Read the model definition and answer for the solid it produces. Units are mm, in the model's axes. Round coordinates to 2 decimals unless told otherwise and drop trailing zeros. Order: outer loops, then holes, each group sorted by start corner. A loop starts at its lowest first (then second) coordinate and runs counter-clockwise, first axis right, second up. Notation, with made-up numbers: (61.25, -15) -> (68.25, -15) arc R12 cw to (68.25, -4) -> close; hole circle Ø5 at (89, 68.25). An arc over 180 degrees is marked (long way). One line per item, written item: value. Start each with the question number.
1. Section D-D (z = 23.5) is taken. Give the vertices of the cut face in (x, y), then the cut area to 3 significant figures.
2. Flat-ended cylindrical pins translate along their axes: pin 1 Ø4 at (x, z) = (31, 16) entering from -Y; pin 2 Ø1 at (x, z) = (14.5, 9.5) entering from -Y; pin 3 Ø4 at (x, z) = (48.5, 13) entering from -Y; pin 4 Ø2 at (x, y) = (8, -2) entering from +Z. Find the tip coordinate at first contact, or state that the pin passes through.
3. Section A-A (z = 17.5) is taken. Give the vertices of the cut face in (x, y), then the cut area to 3 significant figures.
4. The mould has two halves that part along Y. Classify faces 1 (the face through (12, 0, 13)), 2 (the face through (17.334, 13.791, 23.872)), 3 (the face through (0, 8, 13)): released by +Y, released by -Y, zero draft, split by the parting line, or undercut.
5. Section C-C (y = -6.75) is taken. Give the vertices of the cut face in (x, z).
6. Section B-B (x = 10) is taken. Give the vertices of the cut face in (y, z).
7. Consider line 1 (Y direction, x = 2.5, z = 14); line 2 (Y direction, x = 51, z = 6.75); line 3 (X direction, y = 6.5, z = 19.75). Determine where each line is inside the solid, lowest interval first.
from build123d import *

# Parameters (mm, degrees)
F1_DEPTH = 25.4
F2_R     = 5.08
F3_R     = 5.08


# Not quite as in the source:
# - a feature names something its author has since deleted; it is built from what else it names


with BuildPart() as f1:
    # F0 (on Top) → F1 (new body)
    with BuildSketch(Plane.XY):
        Polygon((0, 15.24), (0, 0), (24.13, 0), (55.0936062386, -11.4706359327), (30.48, 15.24), align=None)
    extrude(amount=F1_DEPTH)

    # F2
    f2_edges = [f1.edges().sort_by_distance(p)[0] for p in [
        (15.24, 15.24, 25.4),
    ]]
    fillet(f2_edges, radius=F2_R)

    # F3
    f3_edges = [f1.edges().sort_by_distance(p)[0] for p in [
        (15.24, 15.24, 0),
    ]]
    fillet(f3_edges, radius=F3_R)


solid = f1.part
Answer:
1. outline: (0, 0) -> (24.13, 0) -> (55.09, -11.47) -> (31.51, 14.12) -> (0, 14.12) -> close
1. area: 654 mm^2
2. pin 1: y = -3.29
2. pin 2: y = 0
2. pin 3: y = -9.77
2. pin 4: through
3. outline: (0, 0) -> (24.13, 0) -> (55.09, -11.47) -> (30.48, 15.24) -> (0, 15.24) -> close
3. area: 688 mm^2
4. face 1: released by -Y
4. face 2: released by +Y
4. face 3: zero draft
5. outline: (42.35, 0) -> (50.74, 0) -> (50.74, 25.4) -> (42.35, 25.4) -> close
6. outline: (0, 0) -> (10.16, 0) arc R5.08 ccw to (15.24, 5.08) -> (15.24, 20.32) arc R5.08 ccw to (10.16, 25.4) -> (0, 25.4) -> close
7. line 1: 0 to 15.24
7. line 2: -9.95 to -7.03
7. line 3: 0 to 38.53
